```python
from build123d import *

# Parameters (mm, degrees)
F0_W      = 72.7374479175
F0_H      = 135
F1_DEPTH  = 10
F2_R      = 10
F3_W      = 67
F3_H      = 133
F4_DEPTH  = 8
F5_W      = 12.0182400569
F5_H      = 3.036568407
F6_DEPTH  = 25
F7_R      = 3.1730919104
F8_DEPTH  = 12
F9_W      = 2.8348967899
F9_H      = 53.2759986818
F10_DEPTH = 12


# Not quite as in the source:
# - a feature of the source that left no trace in its solid (it failed there, or was rolled back) is left out


with BuildPart() as f1:
    # F0 (on Front) → F1 (new body)
    with BuildSketch(Plane.XZ):
        Rectangle(F0_W, F0_H)
    extrude(amount=F1_DEPTH)

    # F2
    f2_edges = [f1.edges().sort_by_distance(p)[0] for p in [
        (36.368724, -5, 67.5),
        (-36.368724, -5, 67.5),
        (-36.368724, -5, -67.5),
        (36.368724, -5, -67.5),
    ]]
    fillet(f2_edges, radius=F2_R)

    # F3 (on Front) → F4 (cut)
    with BuildSketch(Plane.XZ):
        Rectangle(F3_W, F3_H)
    extrude(amount=F4_DEPTH, mode=Mode.SUBTRACT)

    # F5 (on face) → F6 (cut)
    with BuildSketch(Plane(origin=(0, 0, -67.5), x_dir=(1, 0, 0), z_dir=(0, 0, -1))):
        with Locations((-18.9633578993, 5.0012452994)):
            Rectangle(F5_W, F5_H)
    extrude(amount=-F6_DEPTH, mode=Mode.SUBTRACT)

    # F7 (on face) → F8 (cut)
    with BuildSketch(Plane.XY.offset(67.5)):
        with Locations((-14.315456152, -4.6320809051)):
            Circle(F7_R)
    extrude(amount=-F8_DEPTH, mode=Mode.SUBTRACT)

    # F9 (on face) → F10 (cut)
    with BuildSketch(Plane(origin=(-36.3687239587, 0, 0), x_dir=(0, -1, 0), z_dir=(-1, 0, 0))):
        with Locations((4.099019221, 26.6379993409)):
            Rectangle(F9_W, F9_H)
    extrude(amount=-F10_DEPTH, mode=Mode.SUBTRACT)


solid = f1.part
```
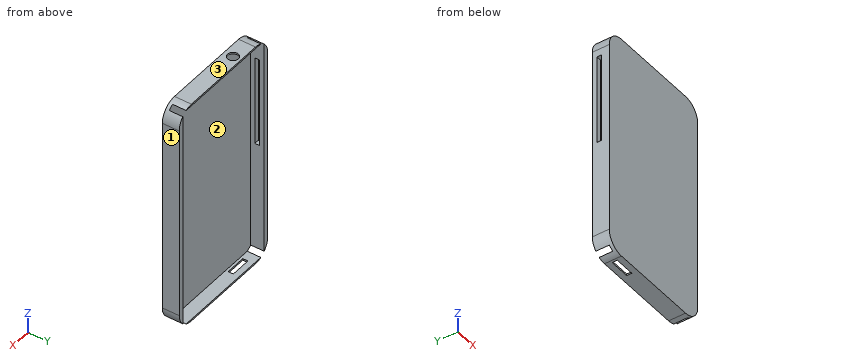
Read the model definition and answer for the solid it produces. Units are mm, in the model's axes. Face numbers are marked on the shaded views. Give positions to 0.01 mm unless a question says otherwise; leave off trailing zeros. Write each loop counter-clockwise with the first axis right and the second up, starting at its lowest first coordinate (ties: lowest second). Pieces come first, ordered by that corner, then holes. Notation, with made-up numbers: (6.5, 28) -> (54.5, 28) arc R28 ccw to (54.5, 47) -> close; hole circle Ø5 at (43.25, 71.5). An arc over 180 degrees is marked (long way). Answer as a JSON object with one key per item and string values.
1) Flat-ended cylindrical pins translate along their axes: pin 1 Ø6 at (x, z) = (-1.5, -18.5) entering from +Y; pin 2 Ø1.1 at (y, z) = (-5.5, -67) entering from +X; pin 3 Ø4 at (x, y) = (-13, -4.5) entering from -Z; pin 4 Ø1.4 at (x, y) = (-34.5, -4) entering from -Z. Find the tip coordinate at first contact, or state that the pin passes through.
Findings below:
{"pin 1": "stops at y = -8", "pin 2": "stops at x = 30.73", "pin 3": "stops at z = -67.5", "pin 4": "stops at z = -64.19"}
2) Straight lines are drawn through the part: probe 1 along X at (y, z) = (-5, -41); probe 2 along Z at (x, y) = (12, -5); probe 3 along Y at (x, z) = (-20, 12). For each, find the intervals that lie inside material, in ascending order. Write a range as from..to.
Findings below:
{"probe 1": "x = -36.37..-33.5, 33.5..36.37", "probe 2": "z = -67.5..-66.5, 66.5..67.5", "probe 3": "y = -10..-8"}
3) Section A-A on x = -23.5 is taken. Write down the section's boundary in (y, z).
Findings below:
{"outline": "(-10, -67.5) -> (-6.52, -67.5) -> (-6.52, -66.5) -> (-8, -66.5) -> (-8, 66.5) -> (0, 66.5) -> (0, 67.5) -> (-10, 67.5) -> close; (-3.48, -67.5) -> (0, -67.5) -> (0, -66.5) -> (-3.48, -66.5) -> close"}
4) Section B-B on z = 40 is taken. Write down the section's boundary in (x, y), then the cut area to 3 significant figures.
Findings below:
{"outline": "(-36.37, -10) -> (36.37, -10) -> (36.37, 0) -> (33.5, 0) -> (33.5, -8) -> (-33.5, -8) -> (-33.5, -5.52) -> (-36.37, -5.52) -> close; (-36.37, -2.68) -> (-33.5, -2.68) -> (-33.5, 0) -> (-36.37, 0) -> close", "area": "183 mm^2"}
5) For a pull along Z with two mould halves and no side action, classify the marked faces 1, 2 and 3 as pulls with the +Z half, pulls with the -Z half, needs draft (parallel to the pull), parting line crosses it, or undercut.
Findings below:
{"face 1": "needs draft", "face 2": "undercut", "face 3": "pulls with the +Z half"}
6) Section C-C on x = 7.5 is taken. Write down the section's boundary in (y, z), then the cut area to 3 significant figures.
Findings below:
{"outline": "(-10, -67.5) -> (0, -67.5) -> (0, -66.5) -> (-8, -66.5) -> (-8, 66.5) -> (0, 66.5) -> (0, 67.5) -> (-10, 67.5) -> close", "area": "286 mm^2"}
7) Section D-D on z = -15.5 is taken. Write down the section's boundary in (x, y), then the cut area to 3 significant figures.
Findings below:
{"outline": "(-36.37, -10) -> (36.37, -10) -> (36.37, 0) -> (33.5, 0) -> (33.5, -8) -> (-33.5, -8) -> (-33.5, 0) -> (-36.37, 0) -> close", "area": "191 mm^2"}
